from build123d import *

# Parameters (mm, degrees)
F1_DEPTH = 6.35
F3_DEPTH = 6.351
F5_DEPTH = 6.351


with BuildPart() as f1:
    # F0 (on Top) → F1 (new body)
    with BuildSketch(Plane.XY):
        with BuildLine():
            Line((113.9825, 84.1375), (-113.9825, 84.1375))
            ThreePointArc((-113.9825, 84.1375), (-117.574602, 82.649602), (-119.0625, 79.0575))
            Line((-119.0625, 79.0575), (-119.0625, -79.0575))
            ThreePointArc((-119.0625, -79.0575), (-117.574602, -82.649602), (-113.9825, -84.1375))
            Line((-113.9825, -84.1375), (113.9825, -84.1375))
            ThreePointArc((113.9825, -84.1375), (117.574602, -82.649602), (119.0625, -79.0575))
            Line((119.0625, -79.0575), (119.0625, 79.0575))
            ThreePointArc((119.0625, 79.0575), (117.574602, 82.649602), (113.9825, 84.1375))
        make_face()
    extrude(amount=F1_DEPTH)

    # F2 (on face) → F3 (cut, through all)
    with BuildSketch(Plane.XY.offset(6.35)):
        Polygon((-95.290107, 46.077607), (0, -49.2125), (95.290107, 46.077607), (31.790107, 46.077607), (0, 14.2875), (-31.790107, 46.077607), align=None)
    extrude(amount=-F3_DEPTH, mode=Mode.SUBTRACT)

    # F4 (on face) → F5 (cut, through all)
    with BuildSketch(Plane.XY.offset(6.35)):
        with BuildLine():
            Line((-97.011982, 46.003431), (-0.556776, -50.451775))
            ThreePointArc((-0.556776, -50.451775), (0, -50.682399), (0.556776, -50.451775))
            Line((0.556776, -50.451775), (97.011982, 46.003431))
            ThreePointArc((97.011982, 46.003431), (97.182669, 46.861532), (96.455206, 47.347607))
            Line((96.455206, 47.347607), (31.590207, 47.347607))
            ThreePointArc((31.590207, 47.347607), (31.288882, 47.287669), (31.033431, 47.116983))
            Line((31.033431, 47.116983), (0.556776, 16.640327))
            ThreePointArc((0.556776, 16.640327), (0, 16.409703), (-0.556776, 16.640327))
            Line((-0.556776, 16.640327), (-31.033431, 47.116983))
            ThreePointArc((-31.033431, 47.116983), (-31.288882, 47.287669), (-31.590207, 47.347607))
            Line((-31.590207, 47.347607), (-96.455206, 47.347607))
            ThreePointArc((-96.455206, 47.347607), (-97.182669, 46.861532), (-97.011982, 46.003431))
        make_face()
    extrude(amount=-F5_DEPTH, mode=Mode.SUBTRACT)


solid = f1.part
Could you check a few things on this model? Use its own coordinates, in mm. A direction names the side the tool comes from. Give positions to 0.01 mm unless a question says otherwise; leave off trailing zeros. Write each loop counter-clockwise with the first axis right and the second up, starting at its lowest first coordinate (ties: lowest second). Pieces come first, ordered by that corner, then holes. Notation, with made-up numbers: (51, 76) - (99, 76) arc R12 cw to (99, 81) - close; hole circle Ø8 at (78.25, -35). An arc over 180 degrees is marked (long way). Use CSV: the item, a comma, the result in double quotes. Start each with the question number.
Item 1: For faces 4 (the face through (117.535, -82.689, 3.131)), 5 (the face through (-15.582, 31.665, 3.219)), which set-ups out of +Z, -Z, +X, -X, +Y, -Y let a thin tool reach every point of the face, with its end or its side?
Item 2: If we mould it in two halves opening along Y, with no side actions, what happens to faces 1 (the face through (-2, 20, 0)), 2 (the face through (-117.614, -82.61, 3.131)), 3 (the face through (16.008, 32.092, 3.219))? For each: pulls with the +Y half, pulls with the -Y half, needs draft (parallel to the pull), parting line crosses it, or undercut.
Item 3: I want a section at A-A, the plane z = 5. Please give me the cut outline in (x, y) (1 decimal).
Item 4: I want a section at B-B, the plane y = -28. Please give me the cut outline in (x, z).
Item 5: I want a section at D-D, the plane y = 19. Please give me the cut outline in (x, z).
Item 6: I want a section at C-C, the plane x = 55. Please give me the cut outline in (y, z), then the cut area to 3 significant figures.
Item 7: If I drill on line 1 along X through (y, z) = (17.5, 4); line 2 along X through (y, z) = (25, 4); line 3 along Y through (x, z) = (87, 3), over which ranges is the centre line in solid material (lowest first)?
Findings:
1,face 4,"+Z, -Z, +X, -Y"
1,face 5,"+Z, -Z"
2,face 1,"needs draft"
2,face 2,"pulls with the -Y half"
2,face 3,"undercut"
3,outline,"(-119.1, -79.1) arc R5.1 ccw to (-114, -84.1) - (114, -84.1) arc R5.1 ccw to (119.1, -79.1) - (119.1, 79.1) arc R5.1 ccw to (114, 84.1) - (-114, 84.1) arc R5.1 ccw to (-119.1, 79.1) - close; hole (-97, 46) - (-0.6, -50.5) arc R0.8 ccw to (0.6, -50.5) - (97, 46) arc R0.8 ccw to (96.5, 47.3) - (31.6, 47.3) arc R0.8 ccw to (31, 47.1) - (0.6, 16.6) arc R0.8 cw to (-0.6, 16.6) - (-31, 47.1) arc R0.8 ccw to (-31.6, 47.3) - (-96.5, 47.3) arc R0.8 ccw to start"
4,outline,"(-119.06, 0) - (-23.01, 0) - (-23.01, 6.35) - (-119.06, 6.35) - close; (23.01, 0) - (119.06, 0) - (119.06, 6.35) - (23.01, 6.35) - close"
5,outline,"(-119.06, 0) - (-70.01, 0) - (-70.01, 6.35) - (-119.06, 6.35) - close; (-2.92, 0) - (2.92, 0) - (2.92, 6.35) - (-2.92, 6.35) - close; (70.01, 0) - (119.06, 0) - (119.06, 6.35) - (70.01, 6.35) - close"
6,outline,"(-84.14, 0) - (3.99, 0) - (3.99, 6.35) - (-84.14, 6.35) - close; (47.35, 0) - (84.14, 0) - (84.14, 6.35) - (47.35, 6.35) - close"
6,area,"793 mm2"
7,line 1,"x = -119.06 to -68.51, -1.42 to 1.42, 68.51 to 119.06"
7,line 2,"x = -119.06 to -76.01, -8.92 to 8.92, 76.01 to 119.06"
7,line 3,"y = -84.14 to 35.99, 47.35 to 84.14"
